Geometry check sheet. Reference: the model listing, model coordinates, mm. Give positions to 0.01 mm unless a question says otherwise; leave off trailing zeros. Loops run counter-clockwise (first coordinate to the right, second up) from the corner with the lowest first, then second, coordinate; pieces in that order, holes last.
```python
from build123d import *

# Parameters (mm, degrees)
SKETCH1_R           = 1.5
BOSS_EXTRUDE1_DEPTH = 1
FILLET2_R           = 5
FILLET3_R           = 5


with BuildPart() as part:
    # Sketch1 → Boss-Extrude1 (new body)
    with BuildSketch(Plane.XY):
        with BuildLine():
            Line((-23.772522595, 48.487733688), (6.227477405, 48.487733688))
            Line((6.227477405, 48.487733688), (6.227477405, 63.487733688))
            ThreePointArc((6.227477405, 63.487733688), (-8.772522595, 78.487733688), (-23.772522595, 63.487733688))
            Line((-23.772522595, 63.487733688), (-23.772522595, 48.487733688))
        make_face()
        with Locations((-14.772522595, 55.987733688)):
            Circle(SKETCH1_R, mode=Mode.SUBTRACT)
        with Locations((-3.272522595, 55.987733688)):
            Circle(SKETCH1_R, mode=Mode.SUBTRACT)
    extrude(amount=BOSS_EXTRUDE1_DEPTH)

    # Fillet2
    fillet2_edges = [part.edges().sort_by_distance(p)[0] for p in [
        (-23.772522595, 48.487733688, 0.5),
    ]]
    fillet(fillet2_edges, radius=FILLET2_R)

    # Fillet3
    fillet3_edges = [part.edges().sort_by_distance(p)[0] for p in [
        (6.227477405, 48.487733688, 0.5),
    ]]
    fillet(fillet3_edges, radius=FILLET3_R)


solid = part.part
```
1) Mould release check, pull along Y, two halves, no side actions. Record for faces 1 (the cylindrical face through (-14.968, 57.475, 0.493)), 2 (the cylindrical face through (-8.443, 78.484, 0.493)), 3 (the flat face through (-9, 64, 1)): +Y half, -Y half, draft (parallel to the pull), parting line (faces both ways), or undercut.
2) Sectioned sample at B-B on y = 74.5. Enter the section's corners in (x, z), plus the area to 3 significant figures.
3) Depth check by flat-ended pin: P1, Ø5, axis at x = -18.5, y = 56.5, coming from the -Z side. Enter the tip coordinate at first touch or a pass-through.
4) Scan lines: line 1 along Y through (x, z) = (-3.5, 0.1); line 2 along Y through (x, z) = (-13.75, 0.8); line 3 along Y through (x, z) = (-5, 0.45). Record each from-to range of solid material in increasing order.
5) Sectioned sample at C-C on x = 0.5. Enter the section's corners in (y, z), plus the area to 3 significant figures.
6) Sectioned sample at A-A on z = 0.35. Enter the section's corners in (x, y).
Determined:
1. face 1: undercut
1. face 2: +Y half
1. face 3: draft
2. outline: (-18.96, 0) - (1.41, 0) - (1.41, 1) - (-18.96, 1) - close
2. area: 20.4 mm2
3. P1: stops at z = 0
4. line 1: y = 48.49 to 54.51, 57.47 to 77.53
4. line 2: y = 48.49 to 54.89, 57.09 to 77.64
4. line 3: y = 48.49 to 78.01
5. outline: (48.49, 0) - (75.28, 0) - (75.28, 1) - (48.49, 1) - close
5. area: 26.8 mm2
6. outline: (-23.77, 53.49) arc R5 ccw to (-18.77, 48.49) - (1.23, 48.49) arc R5 ccw to (6.23, 53.49) - (6.23, 63.49) arc R15 ccw to (-23.77, 63.49) - close; hole circle Ø3 at (-14.77, 55.99); hole circle Ø3 at (-3.27, 55.99)
